from build123d import *

# Parameters (mm, degrees)
SKETCH1_W         = 254
SKETCH1_H         = 206
BODY_DEPTH        = 12.7
SKETCH2_R         = 40
SPIGOT_DEPTH      = 35
SKETCH3_R         = 17.5
HOLE_DEPTH        = 48.7
SLIT_DEPTH        = 0.25
RIGHT_SLITS_COUNT = 5
RIGHT_SLITS_ANGLE = 4
LEFT_SLITS_COUNT  = 9
LEFT_SLITS_ANGLE  = 8
SKETCH7_R         = 0.65
TINY_HOLE_DEPTH   = 0.25


with BuildPart() as part:
    # Sketch1 → Body (new body)
    with BuildSketch(Plane.XY):
        with Locations((0, -3)):
            Rectangle(SKETCH1_W, SKETCH1_H)
    extrude(amount=BODY_DEPTH)

    # Sketch2 → Spigot (add)
    with BuildSketch(Plane.XY.offset(12.7)):
        Circle(SKETCH2_R)
    extrude(amount=SPIGOT_DEPTH)

    # Sketch3 → Hole (cut, through all)
    with BuildSketch(Plane.XY.offset(47.7)):
        Circle(SKETCH3_R)
    extrude(amount=-HOLE_DEPTH, mode=Mode.SUBTRACT)

    # Sketch4 → Slit (cut)
    with BuildSketch(Plane.XY.offset(12.7)):
        Polygon((-117.654454915, 68.216506351), (-107.262150069, 62.216506351), (-107.512150069, 61.783493649), (-117.904454915, 67.783493649), align=None)
    slit = extrude(amount=-SLIT_DEPTH, mode=Mode.SUBTRACT)

    # Right Slits: Slit ×5 about axis
    right_slits_axis = Axis((0, 0, 0), (0, 0, -1))
    for i in range(1, RIGHT_SLITS_COUNT):
        add(slit.rotate(right_slits_axis, i * RIGHT_SLITS_ANGLE / (RIGHT_SLITS_COUNT - 1)), mode=Mode.SUBTRACT)

    # Left Slits: Slit ×9 about axis
    left_slits_axis = Axis((0, 0, 0), (0, 0, 1))
    for i in range(1, LEFT_SLITS_COUNT):
        add(slit.rotate(left_slits_axis, i * LEFT_SLITS_ANGLE / (LEFT_SLITS_COUNT - 1)), mode=Mode.SUBTRACT)

    # Sketch7 → Tiny Hole (cut)
    with BuildSketch(Plane.XY.offset(12.7)):
        with Locations((-119.07849302, 68.75)):
            Circle(SKETCH7_R)
    extrude(amount=-TINY_HOLE_DEPTH, mode=Mode.SUBTRACT)


solid = part.part
Work out the finished part from the listing and answer in its coordinate system (mm). A direction names the side the tool comes from. Round coordinates to 2 decimals unless told otherwise and drop trailing zeros. Loops run counter-clockwise (first coordinate to the right, second up) from the corner with the lowest first, then second, coordinate; pieces in that order, holes last. Notation, with made-up numbers: (-8, 72) -> (-2, 72) arc R18 cw to (-2, 85) -> close; hole circle Ø7 at (63.5, 33). An arc over 180 degrees is marked (long way). Use one line per item in the form item = value.
(1) Flat-ended cylindrical pins translate along their axes: P1, Ø12, axis at x = 32.5, z = 31.5, coming from the +Y side; P2, Ø6.5, axis at x = -114, y = 62.5, coming from the +Z side; P3, Ø4, axis at y = -32, z = 28.5, coming from the -X side. Find the tip coordinate at first contact, or state that the pin passes through.
Answer list:
P1 = 29.96
P2 = 12.7
P3 = -26.46
(2) A tool of negligible diameter and unlimited length cuts with its end or side. For faces 5 (the flat face through (-127, -4, 6)), 6 (the flat face through (-113.7, 63, 12.45)), from which of +Z, -Z, +X, -X, +Y, -Y can it reach the whole face along a straight path? Write none if from no direction.
Answer list:
face_5 = +Z, -Z, -X, +Y, -Y
face_6 = +Z
(3) Find section A-A on y = 0. Give the vertices of the cut face in (x, z), then the cut area to 3 significant figures.
Answer list:
outline = (-127, 0) -> (-17.5, 0) -> (-17.5, 47.7) -> (-40, 47.7) -> (-40, 12.7) -> (-127, 12.7) -> close; (17.5, 0) -> (127, 0) -> (127, 12.7) -> (40, 12.7) -> (40, 47.7) -> (17.5, 47.7) -> close
area = 4,360 mm2
(4) For a pull along Y with two mould halves and no side action, classify faces 1 (the flat face through (127, -4, 6)), 2 (the flat face through (-112.6, 65, 12.45)), 3 (the flat face through (-2, 100, 6)), 4 (the flat face through (-111.4, 67, 12.45)) as released by +Y, released by -Y, zero draft, split by the parting line, or undercut.
Answer list:
face_1 = zero draft
face_2 = undercut
face_3 = released by +Y
face_4 = undercut
(5) Find section C-C on z = 3.5. Give the vertices of the cut face in (x, y).
Answer list:
outline = (-127, -106) -> (127, -106) -> (127, 100) -> (-127, 100) -> close; hole circle Ø35 at (0, 0)
(6) Straight lines are drawn through the part: line 1 (Y direction, x = 0, z = 25); line 2 (X direction, y = 0.5, z = 4); line 3 (Z direction, x = -87.5, y = -71). For each, find the intervals that lie inside material, in ascending order.
Answer list:
line_1 = -40 to -17.5, 17.5 to 40
line_2 = -127 to -17.49, 17.49 to 127
line_3 = 0 to 12.7
(7) Find section B-B on x = -0.5. Give the vertices of the cut face in (y, z).
Answer list:
outline = (-106, 0) -> (-17.49, 0) -> (-17.49, 47.7) -> (-40, 47.7) -> (-40, 12.7) -> (-106, 12.7) -> close; (17.49, 0) -> (100, 0) -> (100, 12.7) -> (40, 12.7) -> (40, 47.7) -> (17.49, 47.7) -> close
(8) Find section D-D on y = -36.5. Give the vertices of the cut face in (x, z).
Answer list:
outline = (-127, 0) -> (127, 0) -> (127, 12.7) -> (16.36, 12.7) -> (16.36, 47.7) -> (-16.36, 47.7) -> (-16.36, 12.7) -> (-127, 12.7) -> close
